Verification items for the finished model (mm, model axes). A direction names the side the tool comes from. Give positions to 0.01 mm unless a question says otherwise; leave off trailing zeros. Write each loop counter-clockwise with the first axis right and the second up, starting at its lowest first coordinate (ties: lowest second). Pieces come first, ordered by that corner, then holes. Notation, with made-up numbers: (53.5, 77.25) -> (64.5, 77.25) arc R24 ccw to (64.5, 101.25) -> close; hole circle Ø11 at (33.5, -22.5). An arc over 180 degrees is marked (long way). Write item = value, one per line.
from build123d import *

# Parameters (mm, degrees)
BOSS_EXTRUDE1_DEPTH     = 11
SKETCH2_W               = 21
SKETCH2_H               = 33
BOSS_EXTRUDE2_DEPTH     = 3
SKETCH3_W               = 2
SKETCH3_H               = 4.664590192
SKETCH3_H_2             = 8.385591547
SKETCH3_H_3             = 5.091451809
CUT_EXTRUDE1_DEPTH      = 4
CUT_EXTRUDE2_REACH      = 25.564
SKETCH4_W               = 15.2
SKETCH4_H               = 30
CUT_EXTRUDE3_DEPTH      = 24.563743336
CUT_EXTRUDE3_DEPTH_BACK = 24.563743336
SKETCH4_3_W             = 43.430774682
SKETCH4_3_H             = 55.651594456


with BuildPart() as part:
    # Sketch1 → Boss-Extrude1 (new body)
    with BuildSketch(Plane(origin=(0, 0, 0), x_dir=(1, 0, 0), z_dir=(0, 1, 0))):
        Polygon((10.5, 15), (7.5, 15), (7.5, -15), (-7.5, -15), (-7.5, 15), (-10.5, 15), (-10.5, -18), (10.5, -18), align=None)
    extrude(amount=BOSS_EXTRUDE1_DEPTH)

    # Sketch2 → Boss-Extrude2 (add)
    with BuildSketch(Plane(origin=(0, 11, 0), x_dir=(1, 0, 0), z_dir=(0, 1, 0))):
        with Locations((0, -1.5)):
            Rectangle(SKETCH2_W, SKETCH2_H)
    extrude(amount=-BOSS_EXTRUDE2_DEPTH)

    # Sketch3 → Cut-Extrude1 (cut)
    with BuildSketch(Plane.XZ):
        with Locations((-6.5, 17.332295096)):
            Rectangle(SKETCH3_W, SKETCH3_H)
        with Locations((0, 19.192795774)):
            Rectangle(SKETCH3_W, SKETCH3_H_2)
        with Locations((6.5, 17.545725905)):
            Rectangle(SKETCH3_W, SKETCH3_H_3)
    extrude(amount=-CUT_EXTRUDE1_DEPTH, mode=Mode.SUBTRACT)

    # Cut-Extrude2: up to this face of the body (flat: up to its plane)
    cut_extrude2_end = Plane(part.part.faces().sort_by_distance((0, 8, 0))[0])
    # Sketch4 → Cut-Extrude2 (cut, up to the picked face)
    with BuildSketch(Plane.XZ, mode=Mode.PRIVATE) as cut_extrude2_sk1:
        with Locations((0.1, 0.2)):
            Rectangle(SKETCH4_W, SKETCH4_H)
    cut_extrude2_tool1 = split(extrude(cut_extrude2_sk1.sketch, amount=-CUT_EXTRUDE2_REACH, mode=Mode.PRIVATE), bisect_by=cut_extrude2_end, keep=Keep.BOTH, mode=Mode.PRIVATE)
    add(cut_extrude2_tool1.solids().sort_by(Axis((0.1, 0, 0.2), (0, 1, 0)))[0], mode=Mode.SUBTRACT)

    # Sketch4<3> → Cut-Extrude3 (cut, two sides: drawn at the far end of the back side and taken through both)
    with BuildSketch(Plane.XZ.offset(-CUT_EXTRUDE3_DEPTH_BACK)):
        Rectangle(SKETCH4_3_W, SKETCH4_3_H)
        Polygon((10.3, -14.8), (7.7, -14.8), (-7.5, -14.8), (-7.5, -15), (-10.5, -15), (-10.5, 18), (-7.5, 18), (-7.5, 17.8), (-5.5, 17.8), (-1, 17.8), (1, 17.8), (5.5, 17.8), (7.5, 17.8), (10.3, 17.8), align=None, mode=Mode.SUBTRACT)
    extrude(amount=CUT_EXTRUDE3_DEPTH + CUT_EXTRUDE3_DEPTH_BACK, mode=Mode.SUBTRACT)


solid = part.part
Item 1: Mould release check, pull along X, two halves, no side actions. Record for faces 6 (the flat face through (-9, 5, -15)), 7 (the flat face through (-7.5, 3, 2)), 8 (the flat face through (10.3, 6, 2)), 9 (the flat face through (7.7, 4, 0)): +X half, -X half, draft (parallel to the pull), parting line (faces both ways), or undercut.
Response values:
face_6 = draft
face_7 = undercut
face_8 = +X half
face_9 = undercut
Item 2: Set-up check for faces 1 (the flat face through (1, 6, 17.8)), 2 (the flat face through (5.5, 2, 16)), 3 (the flat face through (9, 0, 1)), 4 (the flat face through (4, 9, -14.8)), 5 (the flat face through (0, 5, 15.2)): record each of +Z, -Z, +X, -X, +Y, -Y from which the full face is reachable in a straight line by a thin tool's end or side.
Response values:
face_1 = +Z, +X, +Y, -Y
face_2 = +Z, -Z, -Y
face_3 = +Z, -Z, +X, -X, -Y
face_4 = -Z, +X, +Y, -Y
face_5 = -Z, -Y
Item 3: Sectioned sample at B-B on z = -1. Record the cut outline in (x, y), then the cut area to 3 significant figures.
Response values:
outline = (-10.5, 0) -> (-7.5, 0) -> (-7.5, 8) -> (7.7, 8) -> (7.7, 0) -> (10.3, 0) -> (10.3, 11) -> (-10.5, 11) -> close
area = 107 mm^2
Item 4: Material ranges on line 1 (X direction, y = 7.5, z = -4.5); line 2 (Y direction, x = 3.25, z = -1); line 3 (Z direction, x = 7.75, y = 6), recorded low to high.
Response values:
line_1 = -10.5 to -7.5, 7.7 to 10.3
line_2 = 8 to 11
line_3 = -14.8 to 17.8
Item 5: Sectioned sample at D-D on y = 5.5. Record the cut outline in (x, z), then the cut area to 3 significant figures.
Response values:
outline = (-10.5, -15) -> (-7.5, -15) -> (-7.5, 15.2) -> (7.7, 15.2) -> (7.7, -14.8) -> (10.3, -14.8) -> (10.3, 17.8) -> (-7.5, 17.8) -> (-7.5, 18) -> (-10.5, 18) -> close
area = 223 mm^2
Item 6: Sectioned sample at C-C on x = 4.5. Record the cut outline in (y, z), then the cut area to 3 significant figures.
Response values:
outline = (0, 15.2) -> (8, 15.2) -> (8, -14.8) -> (11, -14.8) -> (11, 17.8) -> (0, 17.8) -> close
area = 119 mm^2
Item 7: Go/stop test with flat-tipped pins: P1, Ø1, axis at x = -3, z = -2.5, coming from the -Y side; P2, Ø4, axis at x = -1.5, y = 5.5, coming from the -Z side; P3, Ø1, axis at x = 0, z = 16.5, coming from the -Y side. Record where each tip stops, or that it passes through.
Response values:
P1 = 8
P2 = 15.2
P3 = 4
Item 8: Sectioned sample at A-A on y = 2.25. Record the cut outline in (x, z), then the cut area to 3 significant figures.
Response values:
outline = (-10.5, -15) -> (-7.5, -15) -> (-7.5, 18) -> (-10.5, 18) -> close; (-5.5, 15.2) -> (-1, 15.2) -> (-1, 17.8) -> (-5.5, 17.8) -> close; (1, 15.2) -> (5.5, 15.2) -> (5.5, 17.8) -> (1, 17.8) -> close; (7.5, 15.2) -> (7.7, 15.2) -> (7.7, -14.8) -> (10.3, -14.8) -> (10.3, 17.8) -> (7.5, 17.8) -> close
area = 208 mm^2
